Geometry: final body of the model. Coordinates: model frame, mm. Round coordinates to 2 decimals unless told otherwise and drop trailing zeros. Loops run counter-clockwise (first coordinate to the right, second up) from the corner with the lowest first, then second, coordinate; pieces in that order, holes last. Notation, with made-up numbers: M 81.5,14.25 L 111.5,14.25 A38 ccw 111.5,53.25 Z; hole C 6,64.5 d9. An arc over 180 degrees is marked long. Answer as a JSON object with one key per item and string values.
```python
from build123d import *

# Parameters (mm, degrees)
F0_W     = 11
F0_H     = 30
F0_W_2   = 9
F0_H_2   = 28
F1_DEPTH = 2
F2_W     = 9
F2_H     = 28
F3_DEPTH = 1.5


with BuildPart() as f1:
    # F0 (on Top) → F1 (new body)
    with BuildSketch(Plane.XY):
        Rectangle(F0_W, F0_H)
        Rectangle(F0_W_2, F0_H_2, mode=Mode.SUBTRACT)
        Rectangle(F0_W_2, F0_H_2)
    extrude(amount=-F1_DEPTH)

    # F2 (on face) → F3 (join)
    with BuildSketch(Plane.XY):
        Rectangle(F2_W, F2_H)
    extrude(amount=F3_DEPTH)


solid = f1.part
```
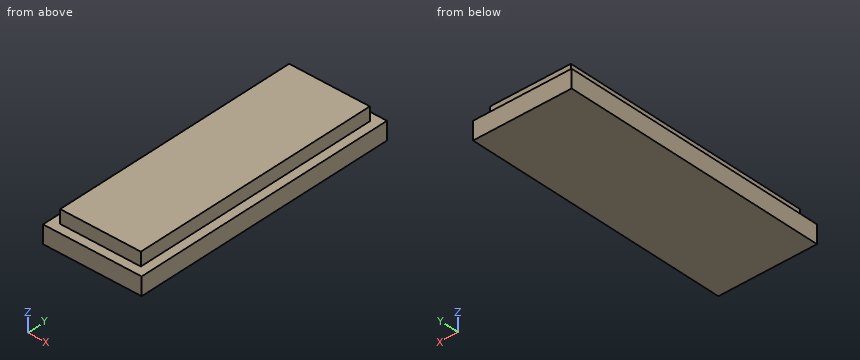
1) Cut plane A-A on y = -0.25. Return the cut outline in (x, z), and give its area (3 significant figures).
Geometry results:
{"outline": "M -5.5,-2 L 5.5,-2 L 5.5,0 L 4.5,0 L 4.5,1.5 L -4.5,1.5 L -4.5,0 L -5.5,0 Z", "area": "35.5 mm2"}
2) Cut plane B-B on x = 2.75. Return the cut outline in (y, z), and give its area (3 significant figures).
Geometry results:
{"outline": "M -15,-2 L 15,-2 L 15,0 L 14,0 L 14,1.5 L -14,1.5 L -14,0 L -15,0 Z", "area": "102 mm2"}
3) First-contact query: pin 1 (0.8 mm diameter, centred on x = 1.5, z = 0.5, fed in from +Y); pin 2 (0.8 mm diameter, centred on y = -3, z = 1, fed in from -X); pin 3 (1.2 mm diameter, centred on y = 7, z = 1, fed in from +X). Flat tips, straight axial feed; report the tip coordinate or a pass-through.
Geometry results:
{"pin 1": "y = 14", "pin 2": "x = -4.5", "pin 3": "x = 4.5"}
4) Line query: probe 1 along Z at (x, y) = (-4.75, -7); probe 2 along X at (y, z) = (4, 0.5); probe 3 along Y at (x, z) = (4, 0.2). Output: solid intervals per line, ascending.
Geometry results:
{"probe 1": "-2 to 0", "probe 2": "-4.5 to 4.5", "probe 3": "-14 to 14"}
